```python
from build123d import *

# Parameters (mm, degrees)
SKETCH1_W          = 130
SKETCH1_H          = 34
SKETCH1_R          = 2.1
SKETCH1_R_2        = 2.15
EXTRUDE1_DEPTH     = 5
EXTRUDE2_DEPTH     = 34
SKETCH4_R          = 4.25
CUT_EXTRUDE1_DEPTH = 34


with BuildPart() as part:
    # Sketch1 → Extrude1 (new body)
    with BuildSketch(Plane.XY):
        with Locations((0, 93.499923245)):
            Rectangle(SKETCH1_W, SKETCH1_H)
        with Locations((35, 93.499923245)):
            Circle(SKETCH1_R, mode=Mode.SUBTRACT)
        with Locations((20, 102.499923245)):
            Circle(SKETCH1_R, mode=Mode.SUBTRACT)
        with Locations((-35, 93.499923245)):
            Circle(SKETCH1_R, mode=Mode.SUBTRACT)
        with Locations((-20, 102.499923245)):
            Circle(SKETCH1_R, mode=Mode.SUBTRACT)
        with Locations((-47.5, 103.499923245)):
            Circle(SKETCH1_R_2, mode=Mode.SUBTRACT)
        with Locations((-47.5, 83.499923245)):
            Circle(SKETCH1_R_2, mode=Mode.SUBTRACT)
        with Locations(Location((47.5, 83.499923245, 0), (0, 0, 180))):
            Circle(SKETCH1_R_2, mode=Mode.SUBTRACT)
        with Locations(Location((47.5, 103.499923245, 0), (0, 0, 180))):
            Circle(SKETCH1_R_2, mode=Mode.SUBTRACT)
    extrude(amount=EXTRUDE1_DEPTH)

    # Sketch3 → Extrude2 (add)
    with BuildSketch(Plane.XZ.offset(-76.499923245)):
        Polygon((-65, 5), (-55.1, 5), (-55.1, 15), align=None)
        Polygon((-39.9, 5), (-19.9, 5), (-39.9, 15), align=None)
        Polygon((39.9, 15), (19.9, 5), (39.9, 5), align=None)
        Polygon((65, 5), (55.1, 15), (55.1, 5), align=None)
    extrude(amount=-EXTRUDE2_DEPTH)

    # Sketch4 → Cut-Extrude1 (cut)
    with BuildSketch(Plane.XY.offset(5)):
        with Locations((-20, 102.499923245)):
            Circle(SKETCH4_R)
        with Locations((19.9, 102.499923245)):
            Circle(SKETCH4_R)
        with Locations((-35, 93.499923245)):
            Circle(SKETCH4_R)
        with Locations(Location((35, 93.499923245, 0), (0, 0, 180))):
            Circle(SKETCH4_R)
    extrude(amount=CUT_EXTRUDE1_DEPTH, mode=Mode.SUBTRACT)


solid = part.part
```
Work out the finished part from the listing and answer in its coordinate system (mm). A direction names the side the tool comes from. Coordinates: 2 decimals unless noted, no trailing zeros. Loops run counter-clockwise (first coordinate to the right, second up) from the corner with the lowest first, then second, coordinate; pieces in that order, holes last. Notation, with made-up numbers: (-8, 29) -> (13, 29) arc R11 ccw to (13, 39) -> close; hole circle Ø10 at (59, 21). An arc over 180 degrees is marked (long way). Answer as CSV lines item,"result".
Q1. The part is cut by section C-C on z = 9.25. Write down the section's boundary in (x, y).
Findings:
outline,"(-60.79, 76.5) -> (-55.1, 76.5) -> (-55.1, 110.5) -> (-60.79, 110.5) -> close; (-39.9, 76.5) -> (-28.4, 76.5) -> (-28.4, 110.5) -> (-39.9, 110.5) -> close; (28.4, 76.5) -> (39.9, 76.5) -> (39.9, 110.5) -> (28.4, 110.5) -> close; (55.1, 76.5) -> (60.79, 76.5) -> (60.79, 110.5) -> (55.1, 110.5) -> close; hole circle Ø8.5 at (-35, 93.5); hole circle Ø8.5 at (35, 93.5)"
Q2. For a pull along X with two mould halves and no side action, classify faces 4 (the face through (-65, 93, 2)), 5 (the face through (-48, 94, 5)), 6 (the face through (-1, 94, 0)) as +X half, -X half, draft (parallel to the pull), parting line (faces both ways), or undercut.
Findings:
face 4,"-X half"
face 5,"undercut"
face 6,"draft"
Q3. The part is cut by section A-A on x = 35. Write down the section's boundary in (y, z), and give its area (3 significant figures).
Findings:
outline,"(76.5, 0) -> (91.4, 0) -> (91.4, 5) -> (89.25, 5) -> (89.25, 12.55) -> (76.5, 12.55) -> close; (95.6, 0) -> (110.5, 0) -> (110.5, 12.55) -> (97.75, 12.55) -> (97.75, 5) -> (95.6, 5) -> close"
area,"342 mm²"
Q4. The part is cut by section B-B on x = -47.5. Write down the section's boundary in (y, z).
Findings:
outline,"(76.5, 0) -> (81.35, 0) -> (81.35, 5) -> (76.5, 5) -> close; (85.65, 0) -> (101.35, 0) -> (101.35, 5) -> (85.65, 5) -> close; (105.65, 0) -> (110.5, 0) -> (110.5, 5) -> (105.65, 5) -> close"
Q5. Find the intervals of material crossed by probe 1 along Y at (x, z) = (-47.5, 1.15); probe 2 along Y at (x, z) = (-35, 10); probe 3 along Y at (x, z) = (-20, 3.2), in increasing order.
Findings:
probe 1,"y = 76.5 to 81.35, 85.65 to 101.35, 105.65 to 110.5"
probe 2,"y = 76.5 to 89.25, 97.75 to 110.5"
probe 3,"y = 76.5 to 100.4, 104.6 to 110.5"
Q6. Each of these flat-tipped pins is pushed along its axis until it touches: pin 1 (7.5 mm diameter, centred on x = 35, y = 93.5, fed in from +Z); pin 2 (3 mm diameter, centred on y = 101.5, z = 7.5, fed in from -X); pin 3 (5 mm diameter, centred on y = 95.5, z = 10, fed in from +X) (3 decimals); pin 4 (4 mm diameter, centred on x = 35, y = 93.5, fed in from +Z). Where does it stop, or does it pass through?
Findings:
pin 1,"stops at z = 5"
pin 2,"stops at x = -64.01"
pin 3,"stops at x = 62.525"
pin 4,"passes through"
Q7. A tool of negligible diameter and unlimited length cuts with its end or side. For faces 1 (the face through (47, 94, 5)), 2 (the face through (46.51, 105.41, 2.46)), 3 (the face through (-37, 95, 5)), from which of +Z, -Z, +X, -X, +Y, -Y can it reach the whole face along a straight path? Write none if from no direction.
Findings:
face 1,"+Z, +Y, -Y"
face 2,"+Z, -Z"
face 3,"+Z"
